Autodesk Fusion 360 part; units mm, degrees
sketch "スケッチ1" plane through (0, 0, 0) normal (0, 0, 1) x (1, 0, 0)
  line L0 (-17.5, 11) -> (17.5, 11)
  line L1 (17.5, 11) -> (17.5, 0)
  line L2 (17.5, 0) -> (-17.5, 0)
  line L3 (-17.5, 0) -> (-17.5, 11)
  dimension "d1" = 35
  dimension "d2" = 11
extrude "押し出し1" add sketch "スケッチ1" along normal blind 120
sketch "スケッチ2" plane through (0, 0, 0) normal (0, 0, -1) x (1, 0, 0)
  line L0 (17.5, 0) -> (-17.5, 0)
  line L1 (-17.5, 0) -> (-17.5, -11)
  line L2 (-17.5, -11) -> (17.5, -11)
  line L3 (17.5, -11) -> (17.5, 0)
  circle A0 centre (0, 0) radius 8.5
  dimension "d5" = 17
extrude "押し出し2" cut sketch "スケッチ2" against normal blind 20 contours L0 A0 picked at (-2.4352, -2.8535)
sketch "スケッチ3" plane through (0, 0, 120) normal (0, 0, 1) x (-1, 0, 0)
  line L0 (17.5, 0) -> (-17.5, 0)
  line L1 (-17.5, 0) -> (-17.5, -11)
  line L2 (-17.5, -11) -> (17.5, -11)
  line L3 (17.5, -11) -> (17.5, 0)
  line L4 (15.5, -9) -> (-15.5, -9)
  line L5 (-15.5, -9) -> (-15.5, 0)
  line L6 (-15.5, 0) -> (15.5, 0)
  line L7 (15.5, 0) -> (15.5, -9)
  dimension "d8" = 2
  dimension "d9" = 31
extrude "押し出し3" cut sketch "スケッチ3" against normal blind 100 contours L0 L4 L5 L6 L7
ref_plane "作業平面1" through (0, 5.5, 9) normal (0, 0, -1) x (-1, 0, 0)
sketch "スケッチ5" plane through (0, 11, 0) normal (0, 1, 0) x (-1, 0, 0)
  line L0 (-17.5, 0) -> (17.5, 0)
  line L1 (17.5, 0) -> (17.5, 120)
  line L2 (17.5, 120) -> (-17.5, 120)
  line L3 (-17.5, 120) -> (-17.5, 0)
  line L4 (-17.5, 130) -> (17.5, 130)
  line L5 (17.5, 130) -> (17.5, 120)
  line L6 (17.5, 120) -> (-17.5, 120)
  line L7 (-17.5, 120) -> (-17.5, 130)
  line L8 (-17.5, 125) -> (17.5, 125) construction
  circle A0 centre (12, 125) radius 2
  circle A1 centre (-12, 125) radius 2
  dimension "d16" = 4
  dimension "d17" = 4
  dimension "d18" = 24
  dimension "d19" = 10
  dimension "d20" = 5.5
extrude "押し出し5" add sketch "スケッチ5" against normal blind 2 contours L2 L4 L5 L6 L7
sketch "スケッチ8" plane through (0, 0, 0) normal (0, -1, 0) x (1, 0, 0)
  line L0 (-8.5, 20) -> (-15.5, 20)
  line L1 (-15.5, 20) -> (-15.5, 120)
  line L2 (-15.5, 120) -> (-17.5, 120)
  line L3 (-17.5, 120) -> (-17.5, 0)
  line L4 (-17.5, 0) -> (-8.5, 0)
  line L5 (-8.5, 0) -> (-8.5, 20)
  circle A0 centre (-14, 15) radius 2.55
  line L6 (18.5, 15) -> (-17.5, 15) construction
  line L7 (17.541, 5) -> (-17.5, 5) construction
  line L8 (15.5, 20) -> (8.5, 20) construction
  circle A1 centre (14, 15) radius 2.55
  circle A2 centre (14, 5) radius 2.55
  circle A3 centre (-14, 5) radius 2.55
  line L9 (17.5, 0) -> (17.5, 120)
  dimension "d30" = 5
  dimension "d31" = 10
  dimension "d32" = 5.1
  dimension "d33" = 5.1
  dimension "d34" = 5.1
  dimension "d35" = 5.1
  dimension "d36" = 3.5
  dimension "d37" = 3.5
  dimension "d38" = 3.5
  dimension "d39" = 3.5
extrude "押し出し8" cut sketch "スケッチ8" against normal blind 15 contours A0 | A1 | A2 | A3
move_face "OffsetFaces1" offset 3 1 faces at (-3.8517, 11, 52.6741)
sketch "Sketch9" plane through (0, 9, 0) normal (0, -1, 0) x (1, 0, 0)
  circle A0 centre (12, 125) radius 2
  circle A1 centre (-12, 125) radius 2
  line L0 (-15.5, 120) -> (-15.5, 20)
  line L1 (-15.5, 20) -> (15.5, 20)
  line L2 (15.5, 20) -> (15.5, 120)
  line L3 (15.5, 120) -> (17.5, 120)
  line L4 (17.5, 120) -> (17.5, 130)
  line L5 (17.5, 130) -> (-17.5, 130)
  line L6 (-17.5, 130) -> (-17.5, 120)
  line L7 (-17.5, 120) -> (-15.5, 120)
  point P0 (12.5, 50)
  point P1 (-12.5, 50)
  point P2 (-12.5, 92)
  point P3 (12.5, 92)
hole "Hole1" at (-12.5, 9, 92) at (12.5, 9, 92) at (12.5, 9, 50) at (-12.5, 9, 50) direction (0, 1, 0) diameter 3.4 depth 9 tip angle 118 countersink diameter 5.6 countersink angle 90
ref_plane "WorkPlane2" through (0, 0, 10) normal (0, 0, 1) x (1, 0, 0)
sketch "Sketch10" plane through (0, 0, 10) normal (0, 0, 1) x (1, 0, 0)
  line L0 (0, 0) -> (15.25, 0)
  line L1 (15.25, 0) -> (15.25, 8)
  line L2 (15.25, 8) -> (0, 10)
  line L3 (0, 0) -> (-15.25, 0)
  line L4 (-15.25, 0) -> (-15.25, 8)
  line L5 (-15.25, 8) -> (0, 10)
  dimension "d60" = 15.25
  dimension "d61" = 8
extrude "Extrude9" cut sketch "Sketch10" along normal blind 0.85 and the other way blind 0.85
sketch "Sketch11" plane through (0, 9, 0) normal (0, -1, 0) x (1, 0, 0)
  circle A0 centre (12.5, 50) radius 2.8
  circle A1 centre (-12.5, 92) radius 2.8
  circle A2 centre (12.5, 92) radius 2.8
  circle A3 centre (-12.5, 50) radius 2.8
  circle A4 centre (-12, 125) radius 2
  circle A5 centre (12, 125) radius 2
  line L0 (-15.5, 120) -> (-15.5, 20)
  line L1 (-15.5, 20) -> (15.5, 20)
  line L2 (15.5, 20) -> (15.5, 120)
  line L3 (15.5, 120) -> (17.5, 120)
  line L4 (17.5, 120) -> (17.5, 130)
  line L5 (17.5, 130) -> (-17.5, 130)
  line L6 (-17.5, 130) -> (-17.5, 120)
  line L7 (-17.5, 120) -> (-15.5, 120)
  line L8 (-17.5, 130) -> (17.5, 130)
  line L9 (17.5, 130) -> (17.5, 120)
  line L10 (17.5, 120) -> (-17.5, 120)
  line L11 (-17.5, 120) -> (-17.5, 130)
extrude "Extrude10" cut sketch "Sketch11" against normal blind 3 contours L3 L4 L5 L6 L7 L8 L9 L10 L11
move_face "OffsetFaces2" offset 2 1 faces at (-3.9094, 14, 64.5049)
move_face "OffsetFaces3" offset 15 1 faces at (5.8333, 13.3333, 130)
sketch "Sketch12" plane through (0, 12, 0) normal (0, -1, 0) x (1, 0, 0)
  circle A0 centre (12, 125) radius 2
  circle A1 centre (-12, 125) radius 2
  line L0 (-17.5, 120) -> (17.5, 120)
  line L1 (17.5, 120) -> (17.5, 145)
  line L2 (17.5, 145) -> (-17.5, 145)
  line L3 (-17.5, 145) -> (-17.5, 120)
  point P0 (-12, 140)
  point P1 (12, 140)
hole "Hole2" at (-12, 12, 140) at (12, 12, 140) direction (0, 1, 0) diameter 4 depth 5 tip angle 118
Read the model definition and answer for the solid it produces. Units are mm, in the model's axes. A direction names the side the tool comes from. Round coordinates to 2 decimals unless told otherwise and drop trailing zeros. Write each loop counter-clockwise with the first axis right and the second up, starting at its lowest first coordinate (ties: lowest second). Pieces come first, ordered by that corner, then holes.
Q1. Find section C-C on z = 5. Determine the outline of the cut face in (x, y).
Values:
outline: (-17.5, 0) - (-16.55, 0) - (-16.55, 16) - (-17.5, 16) - close; (-11.45, 0) - (-8.5, 0) arc R8.5 cw to (8.5, 0) - (11.45, 0) - (11.45, 16) - (-11.45, 16) - close; (16.55, 0) - (17.5, 0) - (17.5, 16) - (16.55, 16) - close
Q2. Straight lines are drawn through the part: line 1 (X direction, y = 14.55, z = 50); line 2 (Z direction, x = 14, y = 6.5); line 3 (X direction, y = 13.8, z = 140). For each, find the intervals that lie inside material, in ascending order.
Values:
line 1: x = -17.5 to -14.2, -10.8 to 10.8, 14.2 to 17.5
line 2: z = 0 to 2.45, 7.55 to 9.15, 10.85 to 12.45, 17.55 to 20
line 3: x = -17.5 to -14, -10 to 10, 14 to 17.5
Q3. Find section B-B on z = 92. Determine the outline of the cut face in (x, y), and give its area (3 significant figures).
Values:
outline: (-17.5, 0) - (-15.5, 0) - (-15.5, 9) - (-15.3, 9) - (-14.2, 10.1) - (-14.2, 16) - (-17.5, 16) - close; (-10.8, 10.1) - (-9.7, 9) - (9.7, 9) - (10.8, 10.1) - (10.8, 16) - (-10.8, 16) - close; (14.2, 10.1) - (15.3, 9) - (15.5, 9) - (15.5, 0) - (17.5, 0) - (17.5, 16) - (14.2, 16) - close
area: 231 mm2
Q4. A tool of negligible diameter and unlimited length cuts with its end or side. For faces 4 (the face through (0, 9, 71)), 5 (the face through (10.925, 14.028, 126.686)), from which of +Z, -Z, +X, -X, +Y, -Y can it reach the whole face along a straight path? Write none if from no direction.
Values:
face 4: +Z, -Y
face 5: +Y, -Y
Q5. Flat-ended cylindrical pins translate along their axes: P1, Ø2, axis at x = -12.5, z = 50, coming from the -Y side; P2, Ø7.5, axis at x = 2.5, z = 130.5, coming from the -Y side; P3, Ø6, axis at x = -5.5, y = 5.5, coming from the +Z side. Find the tip coordinate at first contact, or state that the pin passes through.
Values:
P1: passes through
P2: stops at y = 12
P3: stops at z = 20
Q6. The mould has two halves that part along X. Classify faces 1 (the face through (-12, 14, 142)), 2 (the face through (-1, 10, 120)), 3 (the face through (17.5, 8, 71)): released by +X, released by -X, zero draft, split by the parting line, or undercut.
Values:
face 1: undercut
face 2: zero draft
face 3: released by +X
Q7. Find section A-A on y = 4. Determine the outline of the cut face in (x, z), and give its area (3 significant figures).
Values:
outline: (-17.5, 0) - (-7.5, 0) - (-7.5, 9.15) - (-15.25, 9.15) - (-15.25, 10.85) - (-7.5, 10.85) - (-7.5, 20) - (-15.5, 20) - (-15.5, 120) - (-17.5, 120) - close; (7.5, 0) - (17.5, 0) - (17.5, 120) - (15.5, 120) - (15.5, 20) - (7.5, 20) - (7.5, 10.85) - (15.25, 10.85) - (15.25, 9.15) - (7.5, 9.15) - close; hole circle Ø5.1 at (-14, 5); hole circle Ø5.1 at (-14, 15); hole circle Ø5.1 at (14, 5); hole circle Ø5.1 at (14, 15)
area: 692 mm2
Q8. Find section D-D on z = 33. Determine the outline of the cut face in (x, y), and give its area (3 significant figures).
Values:
outline: (-17.5, 0) - (-15.5, 0) - (-15.5, 9) - (15.5, 9) - (15.5, 0) - (17.5, 0) - (17.5, 16) - (-17.5, 16) - close
area: 281 mm2
